```python
from build123d import *

# Parameters (mm, degrees)
SKETCH1_R           = 9.4262
BOSS_EXTRUDE1_DEPTH = 79.4512
SKETCH2_W           = 3
SKETCH2_H           = 1


with BuildPart() as part:
    # Sketch1 → Boss-Extrude1 (new body)
    with BuildSketch(Plane(origin=(0, 0, 0), x_dir=(0, 0, -1), z_dir=(1, 0, 0))):
        Circle(SKETCH1_R)
        Polygon((7.4203366, 0), (3.7101683, 6.4262), (-3.7101683, 6.4262), (-7.4203366, 0), (-3.7101683, -6.4262), (3.7101683, -6.4262), align=None, mode=Mode.SUBTRACT)
    extrude(amount=BOSS_EXTRUDE1_DEPTH)

    # Sketch2 → Cut-Revolve1 (revolve, cut)
    with BuildSketch(Plane.XY, mode=Mode.PRIVATE) as cut_revolve1_sk:
        with Locations((11.5, 8.9262)):
            Rectangle(SKETCH2_W, SKETCH2_H)
    cut_revolve1 = revolve(cut_revolve1_sk.sketch.rotate(Axis((-1.5494, 0, 0), (1, 0, 0)), 90), axis=Axis((-1.5494, 0, 0), (1, 0, 0)), mode=Mode.SUBTRACT)

    # Mirror1: Cut-Revolve1 across plane
    add(cut_revolve1.mirror(Plane.ZY.offset(-39.7256)), mode=Mode.SUBTRACT)

    # Split1
    split(bisect_by=Plane.ZX, keep=Keep.BOTTOM)


solid = part.part
```
Verification items for the finished model (mm, model axes). A direction names the side the tool comes from. Round coordinates to 2 decimals unless told otherwise and drop trailing zeros. Write each loop counter-clockwise with the first axis right and the second up, starting at its lowest first coordinate (ties: lowest second). Pieces come first, ordered by that corner, then holes.
1. Access from +Z, -Z, +X, -X, +Y, -Y to the whole of each face (thin tool, end or side, straight path). Record for faces 5 (the flat face through (69.451, -9, 0)), 6 (the flat face through (39, -6.426, 0)), 7 (the flat face through (40, 0, -8)).
2. Section check D-D on y = -5.5. Enter the section's corners in (x, z).
3. Section check B-B on z = 0. Enter the section's corners in (x, y).
4. Draft check along Z on faces 1 (the flat face through (39.17, -3.17, 5.59)), 2 (the flat face through (39.17, -3.26, -5.54)), 3 (the flat face through (10, -9, 0)), 4 (the cylindrical face through (11.521, -8.424, 0.185)). Enter one of: +Z half, -Z half, draft (parallel to the pull), parting line (faces both ways), or undercut.
5. Gauge pin test, flat ends, axial feed: P1, Ø5, axis at x = 47, z = 7, coming from the -Y side; P2, Ø3.5, axis at x = 22.5, z = -0.5, coming from the +Y side; P3, Ø1.5, axis at x = 45, y = -1, coming from the -Z side. Record the tip position at first contact, or that the pin passes through.
6. Section check A-A on y = -0.75. Enter the section's corners in (x, z), plus the area to 3 significant figures.
7. Scan lines: L1, parallel to X at y = -8.5, z = -3.75; L2, parallel to Z at x = 43.5, y = -0.5; L3, parallel to Z at x = 34.5, y = -3. Record each from-to range of solid material in increasing order.
8. Section check C-C on x = 23.5. Enter the section's corners in (y, z), plus the area to 3 significant figures.
Answer:
1. face 5: -Y
1. face 6: +X, -X, +Y
1. face 7: +Z, -Z, +X, -X, +Y
2. outline: (0, -7.66) - (10, -7.66) - (10, -6.38) - (13, -6.38) - (13, -7.66) - (66.45, -7.66) - (66.45, -6.38) - (69.45, -6.38) - (69.45, -7.66) - (79.45, -7.66) - (79.45, -4.24) - (0, -4.24) - close; (0, 4.24) - (79.45, 4.24) - (79.45, 7.66) - (69.45, 7.66) - (69.45, 6.38) - (66.45, 6.38) - (66.45, 7.66) - (13, 7.66) - (13, 6.38) - (10, 6.38) - (10, 7.66) - (0, 7.66) - close
3. outline: (0, -9.43) - (10, -9.43) - (10, -8.43) - (13, -8.43) - (13, -9.43) - (66.45, -9.43) - (66.45, -8.43) - (69.45, -8.43) - (69.45, -9.43) - (79.45, -9.43) - (79.45, -6.43) - (0, -6.43) - close
4. face 1: undercut
4. face 2: undercut
4. face 3: draft
4. face 4: parting line
5. P1: stops at y = -8.28
5. P2: stops at y = -6.43
5. P3: stops at z = -9.42
6. outline: (0, -9.4) - (10, -9.4) - (10, -8.39) - (13, -8.39) - (13, -9.4) - (66.45, -9.4) - (66.45, -8.39) - (69.45, -8.39) - (69.45, -9.4) - (79.45, -9.4) - (79.45, -6.99) - (0, -6.99) - close; (0, 6.99) - (79.45, 6.99) - (79.45, 9.4) - (69.45, 9.4) - (69.45, 8.39) - (66.45, 8.39) - (66.45, 9.4) - (13, 9.4) - (13, 8.39) - (10, 8.39) - (10, 9.4) - (0, 9.4) - close
6. area: 371 mm2
7. L1: x = 0 to 10, 13 to 66.45, 69.45 to 79.45
7. L2: z = -9.41 to -7.13, 7.13 to 9.41
7. L3: z = -8.94 to -5.69, 5.69 to 8.94
8. outline: (-6.43, -3.71) - (-6.43, 3.71) - (0, 7.42) - (0, 9.43) arc R9.43 ccw to (0, -9.43) - (0, -7.42) - close
8. area: 68.0 mm2
